Read the model definition and answer for the solid it produces. Units are mm, in the model's axes. Give positions to 0.01 mm unless a question says otherwise; leave off trailing zeros. Write each loop counter-clockwise with the first axis right and the second up, starting at its lowest first coordinate (ties: lowest second). Pieces come first, ordered by that corner, then holes. Notation, with made-up numbers: (6.5, -29.75) -> (44.5, -29.75) arc R7 ccw to (44.5, -17.75) -> close; hole circle Ø6 at (-25.5, -22). An arc over 180 degrees is marked (long way). Answer as CSV lines item,"result". Start each with the question number.
1. The part is cut by section C-C, the plane x = -12. Determine the outline of the cut face in (y, z), and give its area (3 significant figures).
2. The part is cut by section A-A, the plane x = 10.5. Determine the outline of the cut face in (y, z).
3. Find the intervals of material crossed by line 1 (Y direction, x = 4, z = 3.65); line 2 (Y direction, x = -18.5, z = 1.45); line 3 (X direction, y = 12, z = 0.85), in increasing order.
4. Given pin 1 (2 mm diameter, centred on x = -5, z = 2.5, fed in from +Y); pin 2 (2 mm diameter, centred on x = -6, z = 2.5, fed in from -Y); pin 3 (1.5 mm diameter, centred on x = 35, z = 1, fed in from -Y); pin 4 (3.5 mm diameter, centred on x = 79.43, y = -36.51, fed in from +Z), each flat-ended and moving along its own axis, determine where each tip first touches the part or whether it passes through.
5. The part is cut by section D-D, the plane z = 3.25. Give the number of separate pieces and of enclosed holes in the cut face, and give its area (3 significant figures).
6. The part is cut by section B-B, the plane y = 15. Determine the outline of the cut face in (x, z).
from build123d import *

# Parameters (mm, degrees)
EXTRUDE_1_DEPTH          = 4
CUT_EXTRUDE_1_DEPTH      = 42
CUT_EXTRUDE_1_DEPTH_BACK = 10
SKETCH_2_R               = 2.75
SKETCH_3_R               = 5
CUT_EXTRUDE_2_DEPTH      = 1.5


with BuildPart() as part:
    # 草图1 → 凸台-拉伸1 (new body)
    with BuildSketch(Plane.XY):
        with BuildLine():
            Line((-72.574116531, 45.487390308), (77.425883469, 45.487390308))
            ThreePointArc((77.425883469, 45.487390308), (84.496951281, 42.558458119), (87.425883469, 35.487390308))
            Line((87.425883469, 35.487390308), (87.425883469, -34.512609692))
            ThreePointArc((87.425883469, -34.512609692), (84.496951281, -41.583677504), (77.425883469, -44.512609692))
            Line((77.425883469, -44.512609692), (-72.574116531, -44.512609692))
            ThreePointArc((-72.574116531, -44.512609692), (-79.645184343, -41.583677504), (-82.574116531, -34.512609692))
            Line((-82.574116531, -34.512609692), (-82.574116531, 35.487390308))
            ThreePointArc((-82.574116531, 35.487390308), (-79.645184343, 42.558458119), (-72.574116531, 45.487390308))
        make_face()
    extrude(amount=EXTRUDE_1_DEPTH)

    # 草图2 → 切除-拉伸1 (cut, two sides: drawn at the far end of the back side and taken through both)
    with BuildSketch(Plane.XY.offset(4).offset(-CUT_EXTRUDE_1_DEPTH_BACK)):
        with Locations((-74.574116531, 37.487390308)):
            Circle(SKETCH_2_R)
        with Locations((-74.574116531, -36.512609692)):
            Circle(SKETCH_2_R)
        with Locations((79.425883469, 37.487390308)):
            Circle(SKETCH_2_R)
        with Locations((79.425883469, -36.512609692)):
            Circle(SKETCH_2_R)
        with BuildLine():
            Line((-60.749662301, -44.512609692), (60.437772164, -44.512609692))
            ThreePointArc((60.437772164, -44.512609692), (32.253211404, -33.835942142), (2.425883469, -29.512609692))
            ThreePointArc((2.425883469, -29.512609692), (-29.983273004, -33.55318593), (-60.749662301, -44.512609692))
        make_face()
        with BuildLine():
            Line((-62.574116531, 45.487390308), (67.425883469, 45.487390308))
            ThreePointArc((67.425883469, 45.487390308), (35.747267057, 34.428061428), (2.425883469, 30.487390308))
            ThreePointArc((2.425883469, 30.487390308), (-30.918540876, 34.328218147), (-62.574116531, 45.487390308))
        make_face()
        with BuildLine():
            Line((87.425883469, 20.487390308), (87.425883469, -19.512609692))
            ThreePointArc((87.425883469, -19.512609692), (76.286181126, -12.242386449), (72.425883469, 0.487390308))
            ThreePointArc((72.425883469, 0.487390308), (76.286181126, 13.217167065), (87.425883469, 20.487390308))
        make_face()
        with BuildLine():
            Line((-82.574116531, 20.487390308), (-82.574116531, -19.512609692))
            ThreePointArc((-82.574116531, -19.512609692), (-71.434414188, -12.242386449), (-67.574116531, 0.487390308))
            ThreePointArc((-67.574116531, 0.487390308), (-71.434414188, 13.217167065), (-82.574116531, 20.487390308))
        make_face()
        with BuildLine():
            Line((-17.574116531, 20), (22.425883469, 20))
            ThreePointArc((22.425883469, 20), (27.425883469, 15), (22.425883469, 10))
            Line((22.425883469, 10), (-17.574116531, 10))
            ThreePointArc((-17.574116531, 10), (-22.574116531, 15), (-17.574116531, 20))
        make_face()
        with BuildLine():
            Line((-17.079364826, 5), (22.920635174, 5))
            ThreePointArc((22.920635174, 5), (27.920635174, 0), (22.920635174, -5))
            Line((22.920635174, -5), (-17.079364826, -5))
            ThreePointArc((-17.079364826, -5), (-22.079364826, 0), (-17.079364826, 5))
        make_face()
        with BuildLine():
            Line((-17.079364826, -10), (22.920635174, -10))
            ThreePointArc((22.920635174, -10), (27.920635174, -15), (22.920635174, -20))
            Line((22.920635174, -20), (-17.079364826, -20))
            ThreePointArc((-17.079364826, -20), (-22.079364826, -15), (-17.079364826, -10))
        make_face()
    extrude(amount=CUT_EXTRUDE_1_DEPTH + CUT_EXTRUDE_1_DEPTH_BACK, mode=Mode.SUBTRACT)

    # 草图3 → 切除-拉伸2 (cut)
    with BuildSketch(Plane.XY.offset(4)):
        with Locations((-74.574116531, 37.487390308)):
            Circle(SKETCH_3_R)
        with Locations((79.425883469, 37.487390308)):
            Circle(SKETCH_3_R)
        with Locations((79.425883469, -36.512609692)):
            Circle(SKETCH_3_R)
        with Locations((-74.574116531, -36.512609692)):
            Circle(SKETCH_3_R)
    extrude(amount=-CUT_EXTRUDE_2_DEPTH, mode=Mode.SUBTRACT)


solid = part.part
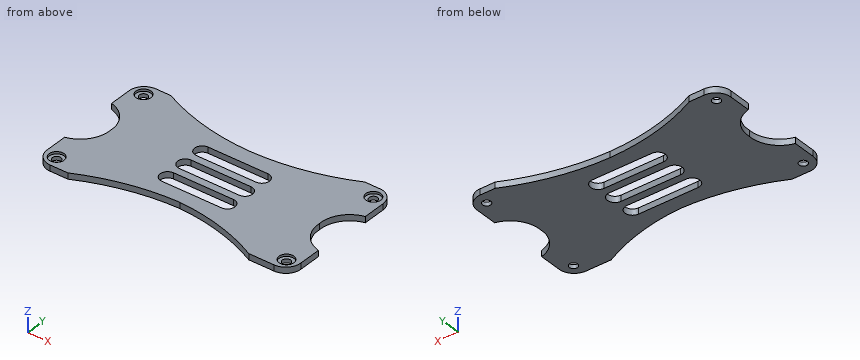
Results found:
1,outline,"(-30.42, 0) -> (-20, 0) -> (-20, 4) -> (-30.42, 4) -> close; (-10, 0) -> (-5, 0) -> (-5, 4) -> (-10, 4) -> close; (5, 0) -> (10, 0) -> (10, 4) -> (5, 4) -> close; (20, 0) -> (31.22, 0) -> (31.22, 4) -> (20, 4) -> close"
1,area,"127 mm²"
2,outline,"(-30.03, 0) -> (-20, 0) -> (-20, 4) -> (-30.03, 4) -> close; (-10, 0) -> (-5, 0) -> (-5, 4) -> (-10, 4) -> close; (5, 0) -> (10, 0) -> (10, 4) -> (5, 4) -> close; (20, 0) -> (30.77, 0) -> (30.77, 4) -> (20, 4) -> close"
3,line 1,"y = -29.58 to -20, -10 to -5, 5 to 10, 20 to 30.51"
3,line 2,"y = -31.3 to -19.79, -10.21 to -4.79, 4.79 to 10.09, 19.91 to 32.01"
3,line 3,"x = -70.59 to -21.57, 26.43 to 75.44"
4,pin 1,"stops at y = 30.75"
4,pin 2,"stops at y = -29.95"
4,pin 3,"stops at y = -34.79"
4,pin 4,"passes through"
5,separate pieces,"1"
5,enclosed holes,"7"
5,area,"10,100 mm²"
6,outline,"(-72.95, 0) -> (-22.57, 0) -> (-22.57, 4) -> (-72.95, 4) -> close; (27.43, 0) -> (77.8, 0) -> (77.8, 4) -> (27.43, 4) -> close"
